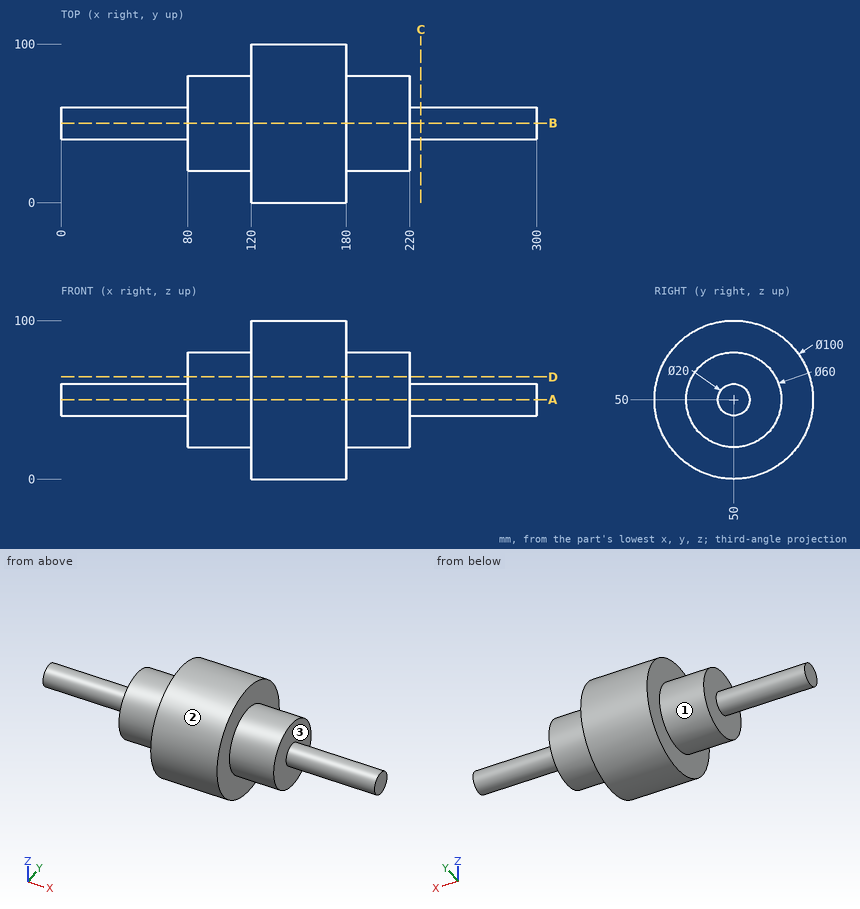
Part print with two shaded views. Sizes in mm from the minimum x, y, z corner. A direction names the side the tool comes from. Coordinates: 2 decimals unless noted, no trailing zeros. Write each loop counter-clockwise with the first axis right and the second up, starting at its lowest first coordinate (ties: lowest second). Pieces come first, ordered by that corner, then holes. Notation, with made-up numbers: (76, 60) -> (88, 60) arc R25 cw to (88, 92) -> close; hole circle Ø8 at (34, 79.25). An arc over 180 degrees is marked (long way). Return JSON: item names as keys, results as strings. Group by question number.
Q1. Cut at A-A, the plane z = 50. Give the cut face in (x, y).
Q2. Drill centre lines: line 1 (X direction, y = 36.5, z = 8.5); line 2 (X direction, y = 33, z = 36); line 3 (Z direction, x = 164, y = 20.5). Where is each one in solid material? Low to high.
Q3. Cut at C-C, the plane x = 227. Give the cut face in (y, z).
Q4. Flat gauge pins, fed straight in: pin 1 (12 mm diameter, centred on x = 234.5, y = 68.5, fed in from +Z); pin 2 (4 mm diameter, centred on x = 96, z = 44, fed in from -Y); pin 3 (2 mm diameter, centred on y = 72.5, z = 90, fed in from -X); pin 4 (4 mm diameter, centred on y = 10.5, z = 29.5, fed in from +X). Where does each tip first touch, or does it go through?
Q5. Cut at D-D, the plane z = 64.5. Give the cut face in (x, y).
Q6. Which spindle directions (+Z, -Z, +X, -X, +Y, -Y) get a long thin tool onto all of the face, cutting with end or side? Do the marked faces 1, 2 and 3. Say none if no direction does.
Returned:
{
 "1": {"outline": "(0, 40) -> (80, 40) -> (80, 20) -> (120, 20) -> (120, 0) -> (180, 0) -> (180, 20) -> (220, 20) -> (220, 40) -> (300, 40) -> (300, 60) -> (220, 60) -> (220, 80) -> (180, 80) -> (180, 100) -> (120, 100) -> (120, 80) -> (80, 80) -> (80, 60) -> (0, 60) -> close"},
 "2": {"line 1": "x = 120 to 180", "line 2": "x = 80 to 220", "line 3": "z = 9.63 to 90.37"},
 "3": {"outline": "circle Ø20 at (50, 50)"},
 "4": {"pin 1": "passes through", "pin 2": "stops at y = 20.27", "pin 3": "stops at x = 120", "pin 4": "stops at x = 180"},
 "5": {"outline": "(80, 23.74) -> (120, 23.74) -> (120, 2.15) -> (180, 2.15) -> (180, 23.74) -> (220, 23.74) -> (220, 76.26) -> (180, 76.26) -> (180, 97.85) -> (120, 97.85) -> (120, 76.26) -> (80, 76.26) -> close"},
 "6": {"face 1": "-X", "face 2": "+X, -X", "face 3": "+X"}
}
